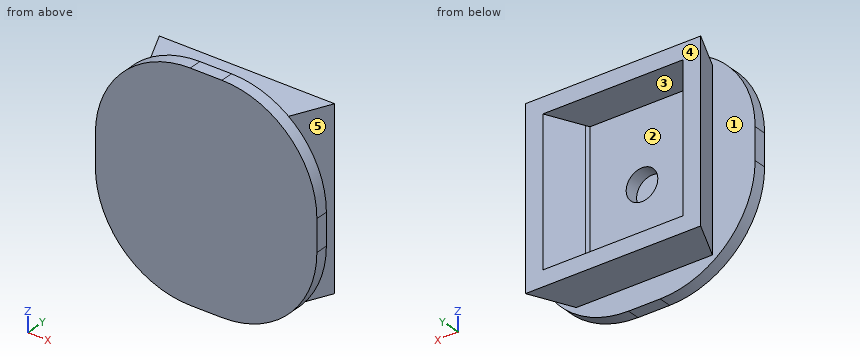
```python
from build123d import *

# Parameters (mm, degrees)
F1_DEPTH     = 6
F3_DEPTH     = 15
F5_DEPTH     = 5.0000008951
F6_R         = 5
F10_DEPTH    = 5
F11_W        = 35
F11_H        = 35
F12_DEPTH    = 2
F15_W        = 27.7
F15_H        = 28
F13_W        = 21.5
F13_H        = 28
F17_T        = 2.5
F17_T3_DEPTH = 26.5
F17_T5_DEPTH = 33
F19_R        = 2.5
F20_DEPTH    = 54.5
F21_R        = 15
F22_R        = 3
F23_R        = 0.5
F24_R        = 2
F25_R        = 6
F28_DEPTH    = 0.3


# Not quite as in the source:
# - ends of sketch curves that miss each other by under 0.0002 mm in the source are joined
# - a shell that OpenCascade refuses in one call is made with other operations: the cavity is built on its own and cut out


with BuildPart() as f1:
    # F0 (on Top) → F1 (new body)
    with BuildSketch(Plane.XY):
        Polygon((11.0000005256, -18.05), (11.0000005256, -20.55), (-11.0000005256, -20.55), (-10.9999994744, 20.55), (11.0000005256, 20.55), (11.0000005256, 18.05), (15.8927322497, 21.8000001848), (16.1137396651, 25.5500003695), (11.4420153564, 25.5500003695), (-15.9999997161, 25.5500003695), (-16.000001023, -25.5500003695), (11.4420153564, -25.5500003695), (16.1137396651, -25.5500003695), (15.8927322497, -21.8000001848), align=None)
    extrude(amount=F1_DEPTH)

    # F2 (on face) → F3 (join)
    with BuildSketch(Plane(origin=(0, 0, 0), x_dir=(1, 0, 0), z_dir=(0, 0, -1))):
        Polygon((-10.9999994744, -25.5500003695), (-15.9999997161, -25.5500003695), (-15.9999997161, -40.5500003695), (-10.9999994744, -40.5500003695), (4.0000002839, -40.5500003695), (4.0000002839, -36.5500003695), (-10.9999994744, -36.5500003695), align=None)
    extrude(amount=-F3_DEPTH)

    # F4 (on face) → F5 (cut, through all)
    with BuildSketch(Plane.YZ.offset(-10.9999994744)):
        Polygon((25.5500003695, 15), (25.5500003695, 6), (29.5500003695, 6), (36.5500003695, 15), align=None)
    extrude(amount=-F5_DEPTH, mode=Mode.SUBTRACT)

    # F6
    f6_edges = [f1.edges().sort_by_distance(p)[0] for p in [
        (4, 38.55, 15),
    ]]
    fillet(f6_edges, radius=F6_R)


with BuildPart() as f10:
    # F9 (on offset) → F10 (new body)
    with BuildSketch(Plane(origin=(0, 65.5500003695, 0), x_dir=(-1, 0, 0), z_dir=(0, 1, 0))):
        with BuildLine():
            Line((15.9999997161, 0), (15.9999997161, 15))
            Line((15.9999997161, 15), (0.9999997161, 15))
            ThreePointArc((0.9999997161, 15), (-2.5355341898, 13.5355339059), (-4.0000002839, 10))
            Line((-4.0000002839, 10), (-4.0000002839, 0))
            Line((-4.0000002839, 0), (15.9999997161, 0))
        make_face()
    extrude(amount=F10_DEPTH)


with BuildPart() as f12:
    # F11 (on offset) → F12 (new body)
    with BuildSketch(Plane(origin=(0, 88.5500003695, 0), x_dir=(-1, 0, 0), z_dir=(0, 1, 0))):
        with Locations((5.9999997161, 7.5)):
            Rectangle(F11_W, F11_H)
    extrude(amount=F12_DEPTH)

    # F15 (on offset) → F16 section 0
    with BuildSketch(Plane(origin=(0, 97.1500003695, 0), x_dir=(-1, 0, 0), z_dir=(0, 1, 0))):
        with Locations((5.9999997161, 7.5)):
            Rectangle(F15_W, F15_H)
    # F13 (on face) → F16 section 1
    with BuildSketch(Plane(origin=(0, 90.5500003695, 0), x_dir=(-1, 0, 0), z_dir=(0, 1, 0))):
        with Locations((5.9999997161, 7.5)):
            Rectangle(F13_W, F13_H)
    loft()

    # F17: shell of thickness 2.5, made by hand


with BuildPart() as f17_core1:
    # F17_t2: copy of F12
    add(f12.part)

    # the walls: a layer under each face that stays
    f17_faces = [f17_core1.faces().sort_by_distance(p)[0] for p in [
        (-5.9999997161, 89.5500003695, -10),
        (11.5000002839, 89.5500003695, 7.5),
        (-23.4999997161, 89.5500003695, 7.5),
        (-5.9999997161, 88.5500003695, 7.5),
        (5.6666669506, 90.5500003695, -4.1666666667),
        (-5.9999997161, 89.5500003695, 25),
        (-5.9999997161, 93.8500003695, -6.5),
        (-18.2999997161, 93.8500003695, 7.5),
        (-5.9999997161, 93.8500003695, 21.5),
        (6.3000002839, 93.8500003695, 7.5),
    ]]
    thicken(f17_faces, amount=-F17_T, mode=Mode.SUBTRACT)

    # F17_s4 → F17_t3 (cut)
    with BuildSketch(Plane.YZ.offset(-19.2499997161)):
        Polygon((90.5750003695, -6.525), (88.0500003695, -6.5), (88.0500003695, -4), (90.5500003695, -4), align=None)
        Polygon((90.5750003695, 21.525), (88.0500003695, 21.5), (88.0500003695, 19), (90.5500003695, 19), align=None)
    extrude(amount=F17_T3_DEPTH, mode=Mode.SUBTRACT)

    # F17_s6 → F17_t5 (cut)
    with BuildSketch(Plane.XY.offset(-9)):
        Polygon((-16.7726279476, 90.5643719578), (-16.7499997161, 88.0500003695), (-12.8137208564, 88.0500003695), (-14.4871765615, 91.6128415482), align=None)
        Polygon((4.7726285154, 90.5643719578), (4.7500002839, 88.0500003695), (0.8137214242, 88.0500003695), (2.4871771293, 91.6128415482), align=None)
    extrude(amount=F17_T5_DEPTH, mode=Mode.SUBTRACT)


with BuildPart() as f12_1:
    add(f12.part)

    # what is left inside the walls is the cavity
    f17_cavity = [f17_core1.part.solids().sort_by_distance(p)[0] for p in [
        (-2.215544, 97.125, 11.243908),
    ]]
    add(f17_cavity, mode=Mode.SUBTRACT)


with BuildPart() as f20_tool:
    # F19 (on face) → F20 (new body, through all)
    with BuildSketch(Plane(origin=(0, 91.0500003695, 0), x_dir=(-1, 0, 0), z_dir=(0, 1, 0))):
        with Locations((5.9999997161, 7.5)):
            Circle(F19_R)
    extrude(amount=-F20_DEPTH)


with BuildPart() as f1_1:
    add(f1.part)

    # F20: cut by f20_tool
    add(f20_tool.part, mode=Mode.SUBTRACT)

    # F22
    f22_edges = [f1_1.edges().sort_by_distance(p)[0] for p in [
        (-16.000001, -25.55, 3),
        (-10.999999, 25.55, 3),
    ]]
    fillet(f22_edges, radius=F22_R)

    # F23
    f23_edges = [f1_1.edges().sort_by_distance(p)[0] for p in [
        (11.000001, -18.05, 3),
        (11.000001, 18.05, 3),
        (-10.999999, 20.55, 3),
        (-11.000001, -20.55, 3),
    ]]
    fillet(f23_edges, radius=F23_R)

    # F24
    f24_edges = [f1_1.edges().sort_by_distance(p)[0] for p in [
        (-16, 40.55, 7.5),
        (-10.999999, 36.55, 7.5),
    ]]
    fillet(f24_edges, radius=F24_R)

    # F25
    f25_edges = [f1_1.edges().sort_by_distance(p)[0] for p in [
        (-13.5, 29.55, 6),
    ]]
    fillet(f25_edges, radius=F25_R)


with BuildPart() as f12_2:
    add(f12_1.part)

    # F20: cut by f20_tool
    add(f20_tool.part, mode=Mode.SUBTRACT)

    # F21
    f21_edges = [f12_2.edges().sort_by_distance(p)[0] for p in [
        (11.5, 89.55, 25),
        (-23.5, 89.55, 25),
        (-23.5, 89.55, -10),
        (11.5, 89.55, -10),
    ]]
    fillet(f21_edges, radius=F21_R)

    # F27 (on face) → F28 (join)
    with BuildSketch(Plane.XZ.offset(-88.5500003695)):
        with BuildLine():
            ThreePointArc((11.5000002839, 10), (7.1066020017, 20.6066017178), (-3.4999997161, 25))
            Line((-3.4999997161, 25), (-8.4999997161, 25))
            ThreePointArc((-8.4999997161, 25), (-19.1066014339, 20.6066017178), (-23.4999997161, 10))
            Line((-23.4999997161, 10), (-23.4999997161, 5))
            ThreePointArc((-23.4999997161, 5), (-19.1066014339, -5.6066017178), (-8.4999997161, -10))
            Line((-8.4999997161, -10), (-3.4999997161, -10))
            ThreePointArc((-3.4999997161, -10), (7.1066020017, -5.6066017178), (11.5000002839, 5))
            Line((11.5000002839, 5), (11.5000002839, 10))
        make_face()
    extrude(amount=-F28_DEPTH)


solid = f12_2.part
```
Work out the finished part from the listing and answer in its coordinate system (mm). Face numbers are marked on the shaded views. A direction names the side the tool comes from. Give positions to 0.01 mm unless a question says otherwise; leave off trailing zeros. Write each loop counter-clockwise with the first axis right and the second up, starting at its lowest first coordinate (ties: lowest second). Pieces come first, ordered by that corner, then holes. Notation, with made-up numbers: (88.5, 52) -> (99.5, 52) arc R13 ccw to (99.5, 74) -> close; hole circle Ø1 at (54, 75). An arc over 180 degrees is marked (long way). Write item = value, one per line.
Q1. Flat-ended cylindrical pins translate along their axes: pin 1 Ø5 at (x, z) = (-6, 6.5) entering from +Y; pin 2 Ø1 at (x, z) = (3, 12) entering from +Y; pin 3 Ø2 at (y, z) = (92, -4) entering from -X. Find the tip coordinate at first contact, or state that the pin passes through.
Computed values:
pin_1 = 91.05
pin_2 = 93.77
pin_3 = -17.9
Q2. Consider line 1 along Z through (x, y) = (2, 92.25); line 2 along Z through (x, y) = (-6, 90.4); line 3 along Y through (x, z) = (-6, -2.5). Determine where each line is inside the solid, lowest interval first.
Computed values:
line_1 = -6.5 to -4, 19 to 21.5
line_2 = -10 to 5, 10 to 25
line_3 = 88.55 to 91.05
Q3. A tool of negligible diameter and unlimited length cuts with its end or side. For the marked faces 3, 4 and 5, from which of +Z, -Z, +X, -X, +Y, -Y can it reach the whole face along a straight path? Write none if from no direction.
Computed values:
face_3 = +Y
face_4 = +Z, -Z, +X, -X, +Y
face_5 = +Z, -Z, +X
Q4. Section B-B on z = 7.5 is taken. Determine the outline of the cut face in (x, y).
Computed values:
outline = (-23.5, 88.55) -> (11.5, 88.55) -> (11.5, 90.55) -> (4.75, 90.55) -> (7.85, 97.15) -> (5.09, 97.15) -> (2.22, 91.05) -> (-3.5, 91.05) -> (-3.5, 88.85) -> (-8.5, 88.85) -> (-8.5, 91.05) -> (-14.22, 91.05) -> (-17.09, 97.15) -> (-19.85, 97.15) -> (-16.75, 90.55) -> (-23.5, 90.55) -> close
Q5. Section A-A on y = 89.5 is taken. Determine the outline of the cut face in (x, z), and give its area (3 significant figures).
Computed values:
outline = (-23.5, 5) arc R15 ccw to (-8.5, -10) -> (-3.5, -10) arc R15 ccw to (11.5, 5) -> (11.5, 10) arc R15 ccw to (-3.5, 25) -> (-8.5, 25) arc R15 ccw to (-23.5, 10) -> close; hole circle Ø5 at (-6, 7.5)
area = 1,010 mm^2
Q6. Section C-C on z = 0.5 is taken. Determine the outline of the cut face in (x, y).
Computed values:
outline = (-22.81, 88.55) -> (10.81, 88.55) -> (10.81, 90.55) -> (4.75, 90.55) -> (7.85, 97.15) -> (5.09, 97.15) -> (2.22, 91.05) -> (-14.22, 91.05) -> (-17.09, 97.15) -> (-19.85, 97.15) -> (-16.75, 90.55) -> (-22.81, 90.55) -> close
Q7. For a pull along Z with two mould halves and no side action, classify the marked faces 1 and 2 as pulls with the +Z half, pulls with the -Z half, needs draft (parallel to the pull), parting line crosses it, or undercut.
Computed values:
face_1 = needs draft
face_2 = undercut
